CAD build for the part. Positions are in the model's coordinates, mm. A direction names the side the tool comes from. Coordinates: 2 decimals unless noted, no trailing zeros. Loops run counter-clockwise (first coordinate to the right, second up) from the corner with the lowest first, then second, coordinate; pieces in that order, holes last. Notation, with made-up numbers: (-21, -34) -> (35, -34) arc R27 ccw to (35, -2) -> close; hole circle Ø5 at (-17.75, 9). An arc over 180 degrees is marked (long way). Write each question's results on one line, items separated by ' | '.
```python
from build123d import *

# Parameters (mm, degrees)
PAD041_DEPTH         = 45
POCKET020_DEPTH      = 55.001
POCKET020_DEPTH_BACK = 55.001
POCKET021_DEPTH      = 8.501


with BuildPart() as part:
    # Sketch123 → Pad041 (new body)
    with BuildSketch(Plane.XY):
        with BuildLine():
            Line((-55, -17.5), (-55, -6))
            ThreePointArc((-53.191343, 0.75), (-54.539999, -2.505943), (-55, -6))
            Line((-53.191343, 0.75), (-47.41784, 10.75))
            ThreePointArc((-35.726497, 17.5), (-42.476497, 15.691343), (-47.41784, 10.75))
            Line((-35.726497, 17.5), (35.726497, 17.5))
            ThreePointArc((47.41784, 10.75), (42.476497, 15.691343), (35.726497, 17.5))
            Line((47.41784, 10.75), (53.191343, 0.75))
            ThreePointArc((55, -6), (54.539999, -2.505943), (53.191343, 0.75))
            Line((55, -6), (55, -17.5))
            ThreePointArc((47.5, -25), (52.803301, -22.803301), (55, -17.5))
            Line((47.5, -25), (-47.5, -25))
            ThreePointArc((-55, -17.5), (-52.803301, -22.803301), (-47.5, -25))
        make_face()
        with BuildLine():
            Line((53.5, -17.5), (53.5, -6))
            ThreePointArc((53.5, -6), (53.09111, -2.894171), (51.892305, 0))
            Line((51.892305, 0), (46.118802, 10))
            ThreePointArc((46.118802, 10), (41.726497, 14.392305), (35.726497, 16))
            Line((35.726497, 16), (-35.726497, 16))
            ThreePointArc((-35.726497, 16), (-41.726497, 14.392305), (-46.118802, 10))
            Line((-46.118802, 10), (-51.892305, 0))
            ThreePointArc((-51.892305, 0), (-53.09111, -2.894171), (-53.5, -6))
            Line((-53.5, -6), (-53.5, -17.5))
            ThreePointArc((-53.5, -17.5), (-51.742641, -21.742641), (-47.5, -23.5))
            Line((-47.5, -23.5), (47.5, -23.5))
            ThreePointArc((47.5, -23.5), (51.742641, -21.742641), (53.5, -17.5))
        make_face(mode=Mode.SUBTRACT)
    extrude(amount=PAD041_DEPTH)

    # Sketch124 → Pocket020 (cut, two sides)
    with BuildSketch(Plane.YZ) as pocket020_sk:
        with BuildLine():
            ThreePointArc((-16, 25), (-11.5, 20.5), (-7, 25))
            ThreePointArc((-4, 25), (-5.5, 26.5), (-7, 25))
            Line((-4, 25), (-4, 20))
            ThreePointArc((-4, 20), (-0.192388, 10.807612), (9, 7))
            Line((9, 50), (9, 7))
            Line((-26.5, 50), (9, 50))
            Line((-26.5, 20.5), (-26.5, 50))
            ThreePointArc((-26.5, 20.5), (-26.06066, 19.43934), (-25, 19))
            ThreePointArc((-25, 19), (-20.757359, 20.757359), (-19, 25))
            ThreePointArc((-16, 25), (-17.5, 26.5), (-19, 25))
        make_face()
    extrude(amount=-POCKET020_DEPTH, mode=Mode.SUBTRACT)
    extrude(pocket020_sk.sketch, amount=POCKET020_DEPTH_BACK, mode=Mode.SUBTRACT)

    # Sketch125 (on DatumPlane) → Pocket021 (cut, through all)
    with BuildSketch(Plane(origin=(0, 9, 7), x_dir=(1, 0, 0), z_dir=(0, -1, 0))):
        with BuildLine():
            ThreePointArc((44, 35.5), (42.347296, 37.469616), (40.120615, 36.18404))
            Line((40.120615, 36.18404), (28.866582, 5.263839))
            ThreePointArc((21.349041, 0), (25.937652, 1.446784), (28.866582, 5.263839))
            Line((-21.349041, 0), (21.349041, 0))
            ThreePointArc((-28.866582, 5.263839), (-25.937652, 1.446784), (-21.349041, 0))
            Line((-40.120615, 36.18404), (-28.866582, 5.263839))
            ThreePointArc((-40.120615, 36.18404), (-42.347296, 37.469616), (-44, 35.5))
            Line((-44, 35.5), (-44, 3))
            ThreePointArc((-47, 0), (-44.87868, 0.87868), (-44, 3))
            Line((-47, 0), (-65, 0))
            ThreePointArc((65, 0), (0, 65), (-65, 0))
            Line((47, 0), (65, 0))
            ThreePointArc((44, 3), (44.87868, 0.87868), (47, 0))
            Line((44, 35.5), (44, 3))
        make_face()
    extrude(amount=-POCKET021_DEPTH, mode=Mode.SUBTRACT)


with BuildPart() as part_1:
    # Body020 placement: moved
    add(part.part.moved(Location((0, 0, 13.3))))


solid = part_1.part
```
Q1. Cut at A-A on x = 3. Write the cut outline in (y, z).
Results are:
outline: (-25, 13.3) -> (-23.5, 13.3) -> (-23.5, 32.49) arc R6 cw to (-25, 32.3) -> close; (16, 13.3) -> (17.5, 13.3) -> (17.5, 20.3) -> (16, 20.3) -> close
Q2. Drop flat-ended pins along their axis: pin 1 (1 mm diameter, centred on y = -4.5, z = 26, fed in from -X); pin 2 (1.7 mm diameter, centred on x = 54, z = 35.5, fed in from +Y); pin 3 (1.1 mm diameter, centred on x = 47.5, y = 10, fed in from +Z). Give the stop position or say it passes through.
Results are:
pin 1: x = -54.96 | pin 2: y = -4 | pin 3: z = 20.3
Q3. Cut at C-C on y = 7.5. Write the cut outline in (x, z).
Results are:
outline: (-49.29, 13.3) -> (-47.56, 13.3) -> (-47.56, 20.39) -> (-49.29, 20.39) -> close; (47.56, 13.3) -> (49.29, 13.3) -> (49.29, 20.39) -> (47.56, 20.39) -> close
Q4. Cut at B-B on z = 18.5. Write the cut outline in (x, y), and give its area (3 significant figures).
Results are:
outline: (-55, -17.5) arc R7.5 ccw to (-47.5, -25) -> (47.5, -25) arc R7.5 ccw to (55, -17.5) -> (55, -6) arc R13.5 ccw to (53.19, 0.75) -> (47.42, 10.75) arc R13.5 ccw to (35.73, 17.5) -> (-35.73, 17.5) arc R13.5 ccw to (-47.42, 10.75) -> (-53.19, 0.75) arc R13.5 ccw to (-55, -6) -> close; hole (-53.5, -17.5) arc R6 ccw to (-47.5, -23.5) -> (47.5, -23.5) arc R6 ccw to (53.5, -17.5) -> (53.5, -6) arc R12 ccw to (51.89, 0) -> (46.12, 10) arc R12 ccw to (35.73, 16) -> (-35.73, 16) arc R12 ccw to (-46.12, 10) -> (-51.89, 0) arc R12 ccw to (-53.5, -6) -> close | area: 411 mm^2
Q5. Wall check: L1, parallel to X at y = -13, z = 23; L2, parallel to Y at x = 28.5, z = 17; L3, parallel to Y at x = 3, z = 24.5. Give the ranges that are in metal, low to high. Write a range as from..to.
Results are:
L1: -55..-53.5, 53.5..55 | L2: -25..-23.5, 16..17.5 | L3: -25..-23.5
Q6. Which spindle directions (+Z, -Z, +X, -X, +Y, -Y) get a long thin tool onto all of the face, cutting with end or side? Do faces 1 (the flat face through (-3, 17.5, 20)), 2 (the flat face through (34.572, 16.576, 41.24)), 3 (the cylindrical face through (-44.9, 12.42, 21.16)), 4 (the cylindrical face through (45.252, 12.424, 20.862)), 5 (the cylindrical face through (53.26, -3.62, 23.43)). Say none if no direction does.
Results are:
face 1: +Z, -Z, +X, -X, +Y | face 2: +Z, +Y | face 3: +Z, -X, +Y | face 4: +Z, +X, +Y | face 5: +Z, -Z
Q7. Pull direction Y, two halves, no side cores. Call faces 6 (the cylindrical face through (-54.2, -11.6, 33.8)), 7 (the cylindrical face through (42.39, 14.7, 57.76)), 8 (the cylindrical face through (-40.983, 16.435, 30.3)): +Y half, -Y half, draft (parallel to the pull), parting line (faces both ways), or undercut.
Results are:
face 6: undercut | face 7: draft | face 8: +Y half
